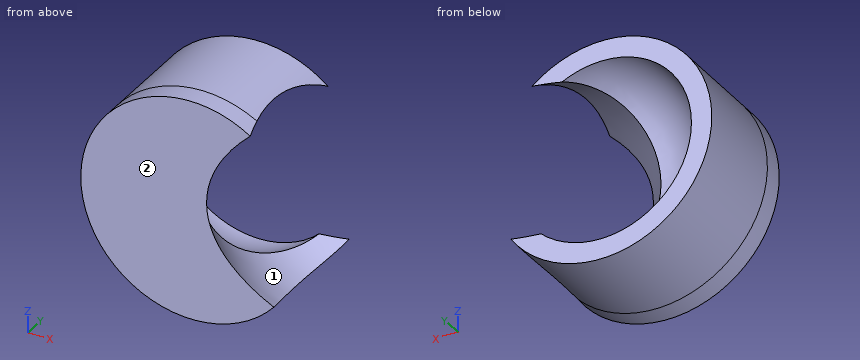
from build123d import *

# Parameters (mm, degrees)
KEYED_BACK_DEPTH   = 0.7
CUP_BLANK_SKETCH_R = 3.8
CUP_BLANK_DEPTH    = 3.3


with BuildPart() as part:
    # Keyed Back Sketch → Keyed Back (new body)
    with BuildSketch(Plane(origin=(0, -97, 0), x_dir=(-1, 0, 0), z_dir=(0, -1, 0))):
        with BuildLine():
            Line((79.27241336, 17.332380758), (79.27241336, 12.667619242))
            ThreePointArc((79.27241336, 12.667619242), (86.07241336, 15), (79.27241336, 17.332380758))
        make_face()
    extrude(amount=KEYED_BACK_DEPTH)

    # Cup Blank Sketch → Cup Blank (add)
    with BuildSketch(Plane(origin=(0, -97.7, 0), x_dir=(-1, 0, 0), z_dir=(0, -1, 0))):
        with Locations(Location((82.27241336, 15, 0), (0, 0, 217.863646362))):
            Circle(CUP_BLANK_SKETCH_R)
    extrude(amount=CUP_BLANK_DEPTH)

    # Spherical Bearing Seat profile → Spherical Bearing Seat (revolve, cut)
    with BuildSketch(Plane(origin=(0, -101, 0), x_dir=(-1, 0, 0), z_dir=(0, -1, 0))):
        with BuildLine():
            Line((82.27241336, 11.9), (82.27241336, 18.1))
            ThreePointArc((82.27241336, 18.1), (79.17241336, 15), (82.27241336, 11.9))
        make_face()
    revolve(axis=Axis((-82.27241336, -101, -25), (0, 0, 1)), mode=Mode.SUBTRACT)

    # Articulation Throat Sketch → Articulation Throat (revolve, cut)
    with BuildSketch(Plane(origin=(21.848129609, -32.292361412, -7.122138515), x_dir=(-0.8343429620590533, -0.5383086561091639, -0.11872494439026368), z_dir=(0.551245699903886, -0.8147619813060819, -0.17969722356136375))):
        Polygon((124.793457491, -7.104979762), (124.793457491, -4.804979762), (101.793457491, 1.915020238), (101.793457491, -7.104979762), align=None)
    revolve(axis=Axis((-90.61584298, -106.383086561, -16.187249444), (0.8343429620590537, 0.5383086561091633, 0.11872494439026321)), mode=Mode.SUBTRACT)


with BuildPart() as body_2:
    # Mirror1: mirrored copy
    add(part.part.mirror(Plane(origin=(0, 0, 0), x_dir=(0, 0, 1), z_dir=(0, -1, 0))))


solid = body_2.part
The listing builds one solid part. Answer for the finished solid, in the listing's coordinates (mm). Face numbers are marked on the shaded views. Give positions to 0.01 mm unless a question says otherwise; leave off trailing zeros. Write each loop counter-clockwise with the first axis right and the second up, starting at its lowest first coordinate (ties: lowest second). Pieces come first, ordered by that corner, then holes.
Item 1: Section A-A, the plane x = -83 is taken. Write down the section's boundary in (y, z), plus the area to 3 significant figures.
Item 2: Find the intervals of material crossed by line 1 along Z through (x, y) = (-83.5, 98.8); line 2 along Z through (x, y) = (-84, 100.6); line 3 along X through (y, z) = (100, -18), in increasing order.
Item 3: Flat-ended cylindrical pins translate along their axes: P1, Ø1, axis at y = 99, z = -16.5, coming from the -X side; P2, Ø1, axis at x = -80, y = 99, coming from the -Z side; P3, Ø2, axis at x = -83.5, z = -14, coming from the +Y side. Find the tip coordinate at first contact, or state that the pin passes through.
Item 4: Determine the mould class of the marked faces 1 and 2 for opening direction Z: released by +Z, released by -Z, zero draft, split by the parting line, or undercut.
Completed:
1. outline: (97, -18.73) - (101, -18.73) - (101, -18.01) arc R3.01 cw to (101, -11.99) - (101, -11.27) - (97, -11.27) - close
1. area: 15.6 mm2
2. line 1: z = -18.6 to -16.81, -13.19 to -11.4
2. line 2: z = -18.38 to -17.54, -12.46 to -11.62
2. line 3: x = -84.6 to -79.94
3. P1: stops at x = -85.94
3. P2: stops at z = -18.36
3. P3: stops at y = 99.29
4. face 1: undercut
4. face 2: zero draft
